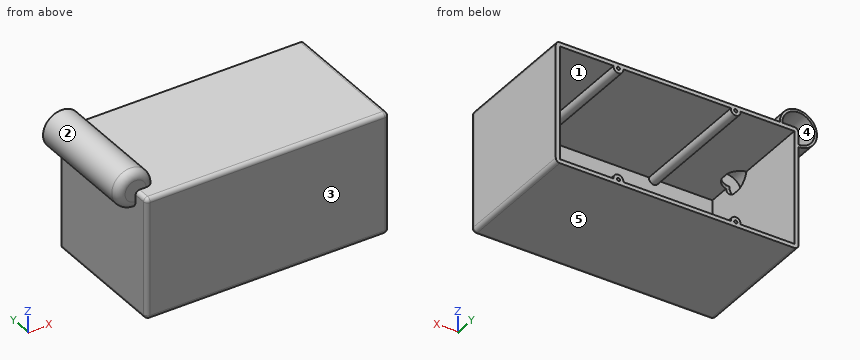
```python
from build123d import *

# Parameters (mm, degrees)
ESQUISSE1_W             = 300
ESQUISSE1_H             = 150
BOSS_EXTRU_1_DEPTH      = 5
ESQUISSE3_W             = 300
ESQUISSE3_H             = 150
ESQUISSE3_W_2           = 290
ESQUISSE3_H_2           = 140
BOSS_EXTRU_2_DEPTH      = 155
ESQUISSE4_R             = 6
BOSS_EXTRU_4_DEPTH      = 155
ESQUISSE5_R             = 1.95
ENL_V_MAT_EXTRU_1_DEPTH = 6
ESQUISSE6_R             = 20
ENL_V_MAT_EXTRU_2_DEPTH = 5
ESQUISSE7_R             = 20
ENL_V_MAT_EXTRU_3_DEPTH = 5
ESQUISSE8_R             = 23
ESQUISSE8_R_2           = 20
BOSS_EXTRU_5_DEPTH      = 140
BOSS_EXTRU_6_START      = -3
ESQUISSE9_R             = 20
BOSS_EXTRU_6_DEPTH      = 3
BOSS_EXTRU_7_DEPTH      = 3
CONG_1_R                = 10
CONG_2_R                = 5
CONG_3_R                = 5
ESQUISSE12_W            = 17.449944321
ESQUISSE12_H            = 17.449944321
ENL_V_MAT_EXTRU_5_DEPTH = 152


# Some blends are built 0.0001 mm under size
with BuildPart() as part:
    # Esquisse1 → Boss.-Extru.1 (new body)
    with BuildSketch(Plane(origin=(0, 0, 0), x_dir=(1, 0, 0), z_dir=(0, 1, 0))):
        Rectangle(ESQUISSE1_W, ESQUISSE1_H)
    extrude(amount=BOSS_EXTRU_1_DEPTH)

    # Esquisse3 → Boss.-Extru.2 (add)
    with BuildSketch(Plane(origin=(0, 5, 0), x_dir=(1, 0, 0), z_dir=(0, 1, 0))):
        Rectangle(ESQUISSE3_W, ESQUISSE3_H)
        Rectangle(ESQUISSE3_W_2, ESQUISSE3_H_2, mode=Mode.SUBTRACT)
    extrude(amount=BOSS_EXTRU_2_DEPTH)

    # Esquisse4 → Boss.-Extru.4 (add)
    with BuildSketch(Plane(origin=(0, 5, 0), x_dir=(1, 0, 0), z_dir=(0, 1, 0))):
        with Locations((-72.5, 69)):
            Circle(ESQUISSE4_R)
        with Locations((72.5, 69)):
            Circle(ESQUISSE4_R)
        with Locations((72.5, -69)):
            Circle(ESQUISSE4_R)
        with Locations((-72.5, -69)):
            Circle(ESQUISSE4_R)
    extrude(amount=BOSS_EXTRU_4_DEPTH)

    # Esquisse5 → Enlèv. mat.-Extru.1 (cut)
    with BuildSketch(Plane(origin=(0, 160, 0), x_dir=(1, 0, 0), z_dir=(0, 1, 0))):
        with Locations(Location((-72.5, 69, 0), (0, 0, 270))):
            Circle(ESQUISSE5_R)
        with Locations(Location((72.5, 69, 0), (0, 0, 90))):
            Circle(ESQUISSE5_R)
        with Locations(Location((72.5, -69, 0), (0, 0, 270))):
            Circle(ESQUISSE5_R)
        with Locations(Location((-72.5, -69, 0), (0, 0, 90))):
            Circle(ESQUISSE5_R)
    extrude(amount=-ENL_V_MAT_EXTRU_1_DEPTH, mode=Mode.SUBTRACT)

    # Esquisse6 → Enlèv. mat.-Extru.2 (cut)
    with BuildSketch(Plane.XY.offset(75)):
        with Locations((-150, 50)):
            Circle(ESQUISSE6_R)
    extrude(amount=-ENL_V_MAT_EXTRU_2_DEPTH, mode=Mode.SUBTRACT)

    # Esquisse7 → Enlèv. mat.-Extru.3 (cut)
    with BuildSketch(Plane.ZY.offset(150)):
        with Locations((75, 50)):
            Circle(ESQUISSE7_R)
    extrude(amount=-ENL_V_MAT_EXTRU_3_DEPTH, mode=Mode.SUBTRACT)

    # Esquisse8 → Boss.-Extru.5 (add)
    with BuildSketch(Plane(origin=(0, 160, 0), x_dir=(1, 0, 0), z_dir=(0, 1, 0))):
        with Locations((-150, -75)):
            Circle(ESQUISSE8_R)
        with Locations((-150, -75)):
            Circle(ESQUISSE8_R_2, mode=Mode.SUBTRACT)
    extrude(amount=-BOSS_EXTRU_5_DEPTH)

    # Esquisse9 → Boss.-Extru.6 (add)
    with BuildSketch(Plane.XZ.offset(-20).offset(BOSS_EXTRU_6_START)):
        with Locations((-150, 75)):
            Circle(ESQUISSE9_R)
    extrude(amount=BOSS_EXTRU_6_DEPTH)

    # Esquisse10 → Boss.-Extru.7 (add)
    with BuildSketch(Plane(origin=(0, 160, 0), x_dir=(1, 0, 0), z_dir=(0, 1, 0))):
        with BuildLine():
            Line((-150, -52), (-150, -75))
            Line((-150, -75), (-127, -75))
            ThreePointArc((-127, -75), (-133.736544033, -58.736544033), (-150, -52))
        make_face()
    extrude(amount=-BOSS_EXTRU_7_DEPTH)

    # Congé1
    cong_1_edges = [part.edges().sort_by_distance(p)[0] for p in [
        (-166.263455967, 20, 91.263455967),
    ]]
    fillet(cong_1_edges, radius=CONG_1_R)

    # Congé2
    cong_2_edges = [part.edges().sort_by_distance(p)[0] for p in [
        (0, 0, -75),
        (150, 0, 0),
        (0, 0, 75),
        (-150, 0, 0),
    ]]
    fillet(cong_2_edges, radius=CONG_2_R - 0.0001)  # a hair under: the kernel refuses the full size

    # Congé3
    # the kernel refuses this fillet: 5 mm, written as the material it takes off along each edge
    with BuildSketch(Plane(origin=(-145, 0, 70), x_dir=(0, 0, 1), z_dir=(1, 0, 0))) as cong_3_piece_1:
        with BuildLine():
            CenterArc((0.0001, -4.9999), 4.9999, 0, 90)
            Line((5, -4.9999), (5, 0))
            Line((5, 0), (0.0001, 0))
        make_face()
    revolve(axis=Axis((-145, 0, 70), (0, -1, 0)), revolution_arc=90, mode=Mode.SUBTRACT)
    with BuildSketch(Plane(origin=(-145, 0, -70), x_dir=(-1, 0, 0), z_dir=(0, 0, 1))) as cong_3_piece_2:
        with BuildLine():
            CenterArc((0.0001, -4.9999), 4.9999, 0, 90)
            Line((5, -4.9999), (5, 0))
            Line((5, 0), (0.0001, 0))
        make_face()
    revolve(axis=Axis((-145, 0, -70), (0, -1, 0)), revolution_arc=90, mode=Mode.SUBTRACT)
    with BuildSketch(Plane(origin=(145, 0, -70), x_dir=(0, 0, -1), z_dir=(-1, 0, 0))) as cong_3_piece_3:
        with BuildLine():
            CenterArc((0.0001, -4.9999), 4.9999, 0, 90)
            Line((5, -4.9999), (5, 0))
            Line((5, 0), (0.0001, 0))
        make_face()
    revolve(axis=Axis((145, 0, -70), (0, -1, 0)), revolution_arc=90, mode=Mode.SUBTRACT)
    with BuildSketch(Plane(origin=(145, 0, 70), x_dir=(1, 0, 0), z_dir=(0, 0, -1))) as cong_3_piece_4:
        with BuildLine():
            CenterArc((0.0001, -4.9999), 4.9999, 0, 90)
            Line((5, -4.9999), (5, 0))
            Line((5, 0), (0.0001, 0))
        make_face()
    revolve(axis=Axis((145, 0, 70), (0, -1, 0)), revolution_arc=90, mode=Mode.SUBTRACT)
    with BuildSketch(Plane(origin=(-150, 20, 75), x_dir=(1, 0, 0), z_dir=(0, -1, 0))) as cong_3_piece_5:
        with BuildLine():
            CenterArc((CONG_3_R, -CONG_3_R), CONG_3_R, 90, 90)
            Line((0, -CONG_3_R), (0, 0))
            Line((0, 0), (CONG_3_R, 0))
        make_face()
    extrude(amount=20, mode=Mode.SUBTRACT)
    with BuildSketch(Plane(origin=(-150, 172.5, 75), x_dir=(1, 0, 0), z_dir=(0, -1, 0))) as cong_3_piece_6:
        with BuildLine():
            CenterArc((CONG_3_R, -CONG_3_R), CONG_3_R, 90, 90)
            Line((0, -CONG_3_R), (0, 0))
            Line((0, 0), (CONG_3_R, 0))
        make_face()
    extrude(amount=115, mode=Mode.SUBTRACT)
    with BuildSketch(Plane(origin=(-150, 172.5, -75), x_dir=(0, 0, 1), z_dir=(0, -1, 0)), Plane(origin=(150, 0, -75), x_dir=(0, 0, 1), z_dir=(0, 1, 0)), Plane(origin=(150, 0, 75), x_dir=(-1, 0, 0), z_dir=(0, 1, 0))) as cong_3_piece_7:
        with BuildLine():
            CenterArc((CONG_3_R, -CONG_3_R), CONG_3_R, 90, 90)
            Line((0, -CONG_3_R), (0, 0))
            Line((0, 0), (CONG_3_R, 0))
        make_face()
    extrude(amount=172.5, mode=Mode.SUBTRACT)

    # Esquisse12 → Enlèv. mat.-Extru.5 (cut)
    with BuildSketch(Plane(origin=(0, 160, 0), x_dir=(1, 0, 0), z_dir=(0, 1, 0))):
        with Locations((-136.27502784, -61.275027839)):
            Rectangle(ESQUISSE12_W, ESQUISSE12_H)
    extrude(amount=-ENL_V_MAT_EXTRU_5_DEPTH, mode=Mode.SUBTRACT)


solid = part.part
```
Geometry: final body of the model. Coordinates: model frame, mm. Face numbers are marked on the shaded views. A direction names the side the tool comes from. Coordinates: 2 decimals unless noted, no trailing zeros. Order: outer loops, then holes, each group sorted by start corner. A loop starts at its lowest first (then second) coordinate and runs counter-clockwise, first axis right, second up. Notation, with made-up numbers: M 63.25,44 L 119.25,44 A12 cw 119.25,59 Z; hole C 50.5,-32 d3. An arc over 180 degrees is marked long. Answer as CSV lines item,"result".
Q1. Line query: probe 1 along X at (y, z) = (158, -69); probe 2 along X at (y, z) = (9.5, -42); probe 3 along Z at (x, y) = (-117.5, 101). Output: solid intervals per line, ascending. Write a range as [from, to].
Answers:
probe 1,"x = [-150, -145], [-78.5, -74.45], [-70.55, -66.5], [66.5, 70.55], [74.45, 78.5], [145, 150]"
probe 2,"x = [-150, -145], [145, 150]"
probe 3,"z = [-75, -70], [70, 75]"
Q2. Section A-A on z = 30. Return the cut outline in (x, y).
Answers:
outline,"M -150,5 A5 ccw -145,0 L 145,0 A5 ccw 150,5 L 150,160 L 145,160 L 145,5 L -145,5 L -145,160 L -150,160 Z"
Q3. Set-up query: the marked faces 4 and 5. Return all of +Z, -Z, +X, -X, +Y, -Y with unobstructed straight access to the full face (end or side cutting, diameter ignored); none if empty.
Answers:
face 4,"+Y"
face 5,"-Z, +X, -X, +Y, -Y"
Q4. Section B-B on x = 96. Return the cut outline in (y, z), and give its area (3 significant figures).
Answers:
outline,"M 0,-70 A5 ccw 5,-75 L 160,-75 L 160,-70 L 5,-70 L 5,70 L 160,70 L 160,75 L 5,75 A5 ccw 0,70 Z"
area,"2,290 mm^2"
Q5. Section D-D on y = 36.5. Return the cut outline in (x, z), and give its area (3 significant figures).
Answers:
outline,"M -150,-70 A5 ccw -145,-75 L 145,-75 A5 ccw 150,-70 L 150,70 A5 ccw 145,75 L -127,75 A23 ccw long -150,52 Z; hole M -150,55 L -150,60.24 L -145,60.24 L -145,-70 L -78.42,-70 A6 cw long -66.58,-70 L 66.58,-70 A6 cw long 78.42,-70 L 145,-70 L 145,70 L 78.42,70 A6 cw long 66.58,70 L -66.58,70 A6 cw long -78.42,70 L -135.24,70 L -135.24,75 L -130,75 A20 ccw long Z"
area,"4,840 mm^2"
Q6. Section C-C on y = 106.5. Return the cut outline in (x, z).
Answers:
outline,"M -150,-70 A5 ccw -145,-75 L 145,-75 A5 ccw 150,-70 L 150,70 A5 ccw 145,75 L -127,75 A23 ccw long -150,52 Z; hole M -150,55 L -150,70 A5 cw -145,75 L -130,75 A20 ccw long Z; hole M -145,-70 L -78.42,-70 A6 cw long -66.58,-70 L 66.58,-70 A6 cw long 78.42,-70 L 145,-70 L 145,70 L 78.42,70 A6 cw long 66.58,70 L -66.58,70 A6 cw long -78.42,70 L -145,70 Z"
Q7. Draft query along X for the marked faces 1, 2 and 3. Return one class per face: pulls with the +X half, pulls with the -X half, needs draft (parallel to the pull), parting line crosses it, or undercut.
Answers:
face 1,"undercut"
face 2,"parting line crosses it"
face 3,"needs draft"
Q8. First-contact query: P1, Ø0.5, axis at x = -148.5, y = 30.5, coming from the +Z side; P2, Ø5, axis at x = 28.5, z = -9.5, coming from the +Y side; P3, Ø12, axis at x = -140.5, y = 124, coming from the +Z side; P4, Ø3, axis at x = 71.5, z = 70, coming from the +Y side. Flat tips, straight axial feed; report the tip coordinate or a pass-through.
Answers:
P1,"stops at z = 97.97"
P2,"stops at y = 5"
P3,"stops at z = 97.73"
P4,"stops at y = 160"
